Autodesk Inventor part; units mm, degrees
ref_plane "YZ Plane" through (0, 0, 0) normal (1, 0, 0) x (0, 1, 0)
ref_plane "XZ Plane" through (0, 0, 0) normal (0, 1, 0) x (-1, 0, 0)
ref_plane "XY Plane" through (0, 0, 0) normal (0, 0, 1) x (1, 0, 0)
sketch "main" plane through (0, 0, 0) normal (0, 0, 1) x (1, 0, 0)
  arc A0 (24.1925, 23.7791) -> (11.4925, 11.0791) centre (24.1925, 11.0791) ccw
  circle A1 centre (11.4925, 30.1291) radius 2.1844
  line L0 (24.1925, 23.7791) -> (24.1925, 23.7791)
  arc A2 (11.4925, 36.4791) -> (6.6143, 34.1942) centre (11.4925, 30.1291) ccw
  circle A3 centre (24.1925, 30.1291) radius 2.1844
  line L1 (24.1925, 36.4791) -> (11.4925, 36.4791)
  arc A4 (24.1925, 23.7791) -> (24.1925, 36.4791) centre (24.1925, 30.1291) ccw
  circle A5 centre (11.4925, -20.6709) radius 2.1844
  circle A6 centre (24.1925, -20.6709) radius 2.1844
  line L2 (24.1925, -14.3081) -> (21.0175, -14.3081)
  arc A7 (24.1539, -27.0337) -> (24.1925, -14.3081) centre (24.1925, -20.6709) ccw
  line L3 (11.4925, 11.0791) -> (11.4925, -4.7831)
  line L4 (6.6143, 34.1942) -> (-25.1357, -3.9059)
  arc A8 (11.4925, -4.7831) -> (21.0175, -14.3081) centre (21.0175, -4.7831) ccw
  circle A9 centre (-20.2575, -7.971) radius 2.0955
  arc A10 (-24.6678, -12.5396) -> (11.5311, -27.0337) centre (11.2178, 24.6342) ccw
  arc A11 (-25.1357, -3.9059) -> (-24.6678, -12.5396) centre (-20.2575, -7.971) ccw
  line L5 (11.5311, -27.0337) -> (24.2311, -27.0337)
  point P0 (10.6662, 5.6616)
  point P1 (11.4925, 23.7791)
  point P2 (11.4925, -14.3081)
  dimension "d0" = 12.7
  dimension "d1" = 12.7
  dimension "d2" = 9.525
sketch "Sketch1" plane through (0, 0, 0) normal (0, 1, 0) x (-1, 0, 0)
  arc A0 (24.1925, 23.7791) -> (11.4925, 11.0791) centre (24.1925, 11.0791) ccw
  circle A1 centre (11.4925, 30.1291) radius 2.1844
  line L0 (24.1925, 23.7791) -> (24.1925, 23.7791)
  arc A2 (11.4925, 36.4791) -> (6.6143, 34.1942) centre (11.4925, 30.1291) ccw
  circle A3 centre (24.1925, 30.1291) radius 2.1844
  line L1 (24.1925, 36.4791) -> (11.4925, 36.4791)
  arc A4 (24.1925, 23.7791) -> (24.1925, 36.4791) centre (24.1925, 30.1291) ccw
  circle A5 centre (11.4925, -20.6709) radius 2.1844
  circle A6 centre (24.1925, -20.6709) radius 2.1844
  line L2 (24.1925, -14.3081) -> (21.0175, -14.3081)
  arc A7 (24.1539, -27.0337) -> (24.1925, -14.3081) centre (24.1925, -20.6709) ccw
  line L3 (11.4925, 11.0791) -> (11.4925, -4.7831)
  line L4 (6.6143, 34.1942) -> (-25.1357, -3.9059)
  arc A8 (11.4925, -4.7831) -> (21.0175, -14.3081) centre (21.0175, -4.7831) ccw
  circle A9 centre (-20.2575, -7.971) radius 2.0955
  arc A10 (-24.6678, -12.5396) -> (11.5311, -27.0337) centre (11.2178, 24.6342) ccw
  arc A11 (-25.1357, -3.9059) -> (-24.6678, -12.5396) centre (-20.2575, -7.971) ccw
  line L5 (11.5311, -27.0337) -> (24.2311, -27.0337)
  point P0 (0, 0)
extrude "Extrusion1" add sketch "Sketch1" along normal blind 1.5875
equation "\"BendRadius\" = Thickness"
equation "\"BendReliefWidth\" = Thickness"
equation "\"BendReliefDepth\" = 0.5 * Thickness"
equation "\"CornerReliefSize\" = 4 * Thickness"
equation "\"MinimumRemnant\" = 2 * Thickness"
equation "\"TransitionRadius\" = BendRadius"
equation "\"JacobiRadiusSize\" = BendRadius"
equation "\"GapSize\" = Thickness"
properties part number "gusset" material "Acetal Resin, White"
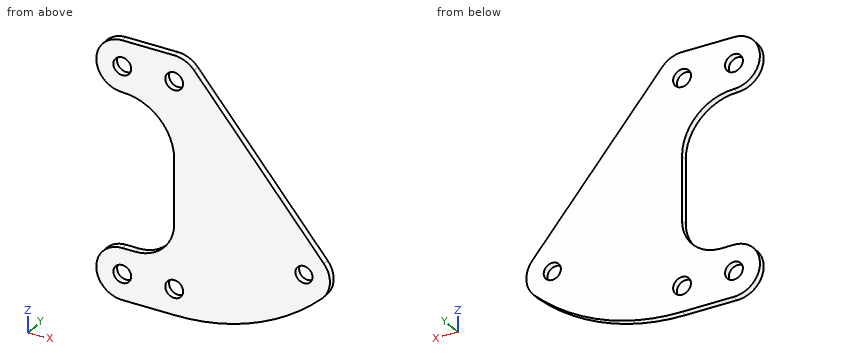
Could you check a few things on this model? Use its own coordinates, in mm. Round coordinates to 2 decimals unless told otherwise and drop trailing zeros. Loops run counter-clockwise (first coordinate to the right, second up) from the corner with the lowest first, then second, coordinate; pieces in that order, holes last.
Q1. For P1, Ø3.5, axis at x = -11.49, z = 30.13, coming from the +Y side, with a flat end and sliding along its axis, tell me the tip position at first contact or that it passes through.
Q2. I want a section at C-C (y = 1.3). Give the number of separate pieces and of enclosed holes in the cut face, and give its area (3 significant figures).
Q3. I want a section at B-B (x = -17.5). Write out the boundary of the cut face in (y, z).
Q4. I want a section at A-A (x = -10). Write out the boundary of the cut face in (y, z).
Q5. I want a section at D-D (z = 5). Write out the boundary of the cut face in (x, y).
Q6. Please list where these lines run through material, in increasing order: L1, parallel to Z at x = -9.5, y = 1.15; L2, parallel to X at y = 1.5, z = 28.5; L3, parallel to Z at x = -10, y = 0.2.
Answer below:
1. P1: passes through
2. separate pieces: 1
2. enclosed holes: 5
2. area: 1,910 mm2
3. outline: (0, -27.03) - (1.59, -27.03) - (1.59, -13.63) - (0, -13.63) - close; (0, 21.87) - (1.59, 21.87) - (1.59, 36.48) - (0, 36.48) - close
4. outline: (0, -27.02) - (1.59, -27.02) - (1.59, -22.27) - (0, -22.27) - close; (0, -19.08) - (1.59, -19.08) - (1.59, 28.53) - (0, 28.53) - close; (0, 31.72) - (1.59, 31.72) - (1.59, 36.3) - (0, 36.3) - close
5. outline: (-11.49, 0) - (17.71, 0) - (17.71, 1.59) - (-11.49, 1.59) - close
6. L1: z = -27.01 to -21.57, -19.78 to 29.23, 31.02 to 36.16
6. L2: x = -30.33 to -25.65, -22.74 to -12.95, -10.04 to -1.87
6. L3: z = -27.02 to -22.27, -19.08 to 28.53, 31.72 to 36.3
